Geometry: final body of the model. Coordinates: model frame, mm. A direction names the side the tool comes from. Coordinates: 2 decimals unless noted, no trailing zeros. Order: outer loops, then holes, each group sorted by start corner. A loop starts at its lowest first (then second) coordinate and runs counter-clockwise, first axis right, second up. Notation, with made-up numbers: M 78,-39.75 L 134,-39.75 A27 cw 134,-1.75 Z; hole C 42,-12 d4. An arc over 180 degrees is marked long. Write item = value, one per line.
from build123d import *

# Parameters (mm, degrees)
F0_R     = 2.1
F1_DEPTH = 16
F2_SIZE  = 2
F4_DEPTH = 3.1
F6_DEPTH = 12
F7_R     = 2
F8_DEPTH = 256.101


with BuildPart() as f1:
    # F0 (on Top) → F1 (new body)
    with BuildSketch(Plane.XY):
        with BuildLine():
            Line((174.5, 129), (-174.5, 129))
            ThreePointArc((-174.5, 129), (-182.985281, 125.485281), (-186.5, 117))
            Line((-186.5, 117), (-186.5, -117))
            ThreePointArc((-186.5, -117), (-182.985281, -125.485281), (-174.5, -129))
            Line((-174.5, -129), (174.5, -129))
            ThreePointArc((174.5, -129), (182.985281, -125.485281), (186.5, -117))
            Line((186.5, -117), (186.5, 117))
            ThreePointArc((186.5, 117), (182.985281, 125.485281), (174.5, 129))
        make_face()
        with Locations((-166.5, -64)):
            Circle(F0_R, mode=Mode.SUBTRACT)
        with Locations((166.5, -64)):
            Circle(F0_R, mode=Mode.SUBTRACT)
        with Locations((-166.5, 64)):
            Circle(F0_R, mode=Mode.SUBTRACT)
        with BuildLine():
            ThreePointArc((-171.5, 109), (-170.035534, 112.535534), (-166.5, 114))
            Line((-166.5, 114), (166.5, 114))
            ThreePointArc((166.5, 114), (170.035534, 112.535534), (171.5, 109))
            Line((171.5, 109), (171.5, 72))
            Line((171.5, 72), (154.5, 72))
            Line((154.5, 72), (154.5, 56))
            Line((154.5, 56), (171.5, 56))
            Line((171.5, 56), (171.5, -56))
            Line((171.5, -56), (154.5, -56))
            Line((154.5, -56), (154.5, -72))
            Line((154.5, -72), (171.5, -72))
            Line((171.5, -72), (171.5, -109))
            ThreePointArc((171.5, -109), (170.035534, -112.535534), (166.5, -114))
            Line((166.5, -114), (-166.5, -114))
            ThreePointArc((-166.5, -114), (-170.035534, -112.535534), (-171.5, -109))
            Line((-171.5, -109), (-171.5, -72))
            Line((-171.5, -72), (-154.5, -72))
            Line((-154.5, -72), (-154.5, -56))
            Line((-154.5, -56), (-171.5, -56))
            Line((-171.5, -56), (-171.5, 56))
            Line((-171.5, 56), (-154.5, 56))
            Line((-154.5, 56), (-154.5, 72))
            Line((-154.5, 72), (-171.5, 72))
            Line((-171.5, 72), (-171.5, 109))
        make_face(mode=Mode.SUBTRACT)
        with Locations((166.5, 64)):
            Circle(F0_R, mode=Mode.SUBTRACT)
    extrude(amount=F1_DEPTH)

    # F2
    f2_edges = [f1.edges().sort_by_distance(p)[0] for p in [
        (0, -129, 16),
    ]]
    chamfer(f2_edges, length=F2_SIZE)

    # F3 (on face) → F4 (cut)
    with BuildSketch(Plane.XY.offset(16)):
        with BuildLine():
            ThreePointArc((-174.5, 125), (-180.156854, 122.656854), (-182.5, 117))
            Line((-182.5, 117), (-182.5, -117))
            ThreePointArc((-182.5, -117), (-180.156854, -122.656854), (-174.5, -125))
            Line((-174.5, -125), (174.5, -125))
            ThreePointArc((174.5, -125), (180.156854, -122.656854), (182.5, -117))
            Line((182.5, -117), (182.5, 117))
            ThreePointArc((182.5, 117), (180.156854, 122.656854), (174.5, 125))
            Line((174.5, 125), (-174.5, 125))
        make_face()
    extrude(amount=-F4_DEPTH, mode=Mode.SUBTRACT)

    # F5 (on face) → F6 (cut)
    with BuildSketch(Plane.XY):
        with BuildLine():
            Line((172.6, 132.1), (-172.6, 132.1))
            ThreePointArc((-172.6, 132.1), (-184.620815, 127.120815), (-189.6, 115.1))
            Line((-189.6, 115.1), (-189.6, -115.1))
            ThreePointArc((-189.6, -115.1), (-184.620815, -127.120815), (-172.6, -132.1))
            Line((-172.6, -132.1), (172.6, -132.1))
            ThreePointArc((172.6, -132.1), (184.620815, -127.120815), (189.6, -115.1))
            Line((189.6, -115.1), (189.6, 115.1))
            ThreePointArc((189.6, 115.1), (184.620815, 127.120815), (172.6, 132.1))
        make_face()
        with BuildLine():
            ThreePointArc((-184.6, 115.1), (-181.085281, 123.585281), (-172.6, 127.1))
            Line((-172.6, 127.1), (172.6, 127.1))
            ThreePointArc((172.6, 127.1), (181.085281, 123.585281), (184.6, 115.1))
            Line((184.6, 115.1), (184.6, -115.1))
            ThreePointArc((184.6, -115.1), (181.085281, -123.585281), (172.6, -127.1))
            Line((172.6, -127.1), (-172.6, -127.1))
            ThreePointArc((-172.6, -127.1), (-181.085281, -123.585281), (-184.6, -115.1))
            Line((-184.6, -115.1), (-184.6, 115.1))
        make_face(mode=Mode.SUBTRACT)
    extrude(amount=F6_DEPTH, mode=Mode.SUBTRACT)

    # F7 (on face) → F8 (cut, through all)
    with BuildSketch(Plane.XZ.offset(127.1)):
        with Locations((-163, 8)):
            Circle(F7_R)
        with Locations((163, 8)):
            Circle(F7_R)
    extrude(amount=-F8_DEPTH, mode=Mode.SUBTRACT)


solid = f1.part
1) Line query: L1, parallel to Y at x = 25, z = 8.25; L2, parallel to Z at x = 163, y = 124.5; L3, parallel to X at y = -21, z = 9.5. Output: solid intervals per line, ascending.
Numbers:
L1 = -127.1 to -114, 114 to 127.1
L2 = 0 to 6, 10 to 12.9
L3 = -184.6 to -171.5, 171.5 to 184.6
2) Pin query (flat end, axial travel): pin 1 (8 mm diameter, centred on y = 30.5, z = 2, fed in from -X); pin 2 (3.5 mm diameter, centred on x = 16.5, z = 8.5, fed in from +Y); pin 3 (2.5 mm diameter, centred on x = 163, z = 8, fed in from -Y); pin 4 (6.5 mm diameter, centred on y = -87.5, z = 6, fed in from +X). Return the tip coordinate at first contact, or that it passes through.
Numbers:
pin_1 = -184.6
pin_2 = 127.1
pin_3 = through
pin_4 = 184.6
3) Mould query, pull axis Y, two halves, no side actions, for faces 4 (the face through (171.5, -90, 6)), 5 (the face through (182.036, 124.372, 15.458)), 6 (the face through (2, -127.1, 6)), 7 (the face through (-154.5, -64, 6)). Classes: pulls with the +Y half, pulls with the -Y half, needs draft (parallel to the pull), parting line crosses it, or undercut.
Numbers:
face_4 = undercut
face_5 = pulls with the +Y half
face_6 = pulls with the -Y half
face_7 = undercut
4) Section A-A, the plane x = 76. Return loops of the section in (y, z).
Numbers:
outline = M -129,12 L -127.1,12 L -127.1,0 L -114,0 L -114,12.9 L -125,12.9 L -125,16 L -127,16 L -129,14 Z; M 114,0 L 127.1,0 L 127.1,12 L 129,12 L 129,14 L 127,16 L 125,16 L 125,12.9 L 114,12.9 Z
5) Set-up query: faces 1 (the face through (184.6, 2, 6)), 2 (the face through (-180.99, -123.68, 5.92)), 3 (the face through (-154.5, 64, 6)). Return all of +Z, -Z, +X, -X, +Y, -Y with unobstructed straight access to the full face (end or side cutting, diameter ignored); none if empty.
Numbers:
face_1 = -Z, +X, +Y, -Y
face_2 = -Z, -X, -Y
face_3 = +Z, -Z
6) Section B-B, the plane y = -31.5. Return loops of the section in (x, z).
Numbers:
outline = M -186.5,12 L -184.6,12 L -184.6,0 L -171.5,0 L -171.5,12.9 L -182.5,12.9 L -182.5,16 L -184.5,16 L -186.5,14 Z; M 171.5,0 L 184.6,0 L 184.6,12 L 186.5,12 L 186.5,14 L 184.5,16 L 182.5,16 L 182.5,12.9 L 171.5,12.9 Z
7) Section C-C, the plane z = 3.5. Give the number of separate pieces and of enclosed holes in the cut face, and give its area (3 significant figures).
Numbers:
separate_pieces = 1
enclosed_holes = 5
area = 16,600 mm²
